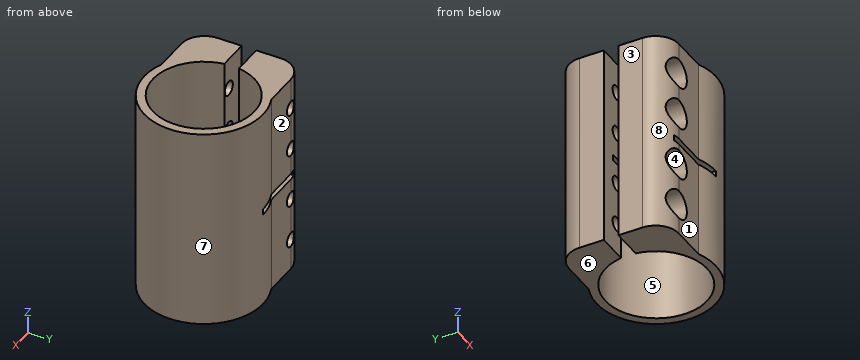
from build123d import *

# Parameters (mm, degrees)
F1_DEPTH       = 35
F3_D           = 5
F3_START       = 1.7550021
F3_CBORE_D     = 10
F3_CBORE_DEPTH = 8
F4_W           = 22.4
F4_H           = 2
F5_DEPTH       = 25


with BuildPart() as f1:
    # F0 (on Top) → F1 (new body, symmetric)
    with BuildSketch(Plane.XY):
        with BuildLine():
            ThreePointArc((-17.3192642082, 2.5086026559), (17.5, 0), (-17.3192642082, -2.5086026559))
            Line((-17.3192642082, -2.5086026559), (-28.1192642082, -2.5086026559))
            Line((-28.1192642082, -2.5086026559), (-28.1192642082, -10.9086026559))
            ThreePointArc((-28.1192642082, -10.9086026559), (-25.7761184577, -16.5654569054), (-20.1192642082, -18.9086026559))
            Line((-20.1192642082, -18.9086026559), (-7.9192642082, -18.9086026559))
            ThreePointArc((-7.9192642082, -18.9086026559), (20.5, 0), (-7.9192642082, 18.9086026559))
            Line((-7.9192642082, 18.9086026559), (-20.1192642082, 18.9086026559))
            ThreePointArc((-20.1192642082, 18.9086026559), (-25.7761184577, 16.5654569054), (-28.1192642082, 10.9086026559))
            Line((-28.1192642082, 10.9086026559), (-28.1192642082, 2.5086026559))
            Line((-28.1192642082, 2.5086026559), (-17.3192642082, 2.5086026559))
        make_face()
    extrude(amount=F1_DEPTH, both=True)

    # F3 (through all)
    # its depths count from where the whole tool has entered the part; down to there all is cleared
    with Locations(Plane.XZ.offset(18.9086026559).offset(-F3_START)):
        with Locations((-20.1192642082, 24.25), (-20.1192642082, 9.25), (-20.1192642082, -9.25), (-20.1192642082, -24.25)):
            CounterBoreHole(F3_D / 2, F3_CBORE_D / 2, F3_CBORE_DEPTH)

    # F4 (on Front) → F5 (cut, symmetric)
    with BuildSketch(Plane.XZ):
        with Locations((-11.2, -1)):
            Rectangle(F4_W, F4_H)
    extrude(amount=F5_DEPTH, both=True, mode=Mode.SUBTRACT)


solid = f1.part
Source: CAD feature listing. Evaluate the final solid. Frame: model axes, mm. Face numbers are marked on the shaded views. A direction names the side the tool comes from. Round coordinates to 2 decimals unless told otherwise and drop trailing zeros. Loops run counter-clockwise (first coordinate to the right, second up) from the corner with the lowest first, then second, coordinate; pieces in that order, holes last.
Q1. Ray query, line 1 (Y direction, x = 0, z = 26.5); line 2 (Z direction, x = -4, y = 19); line 3 (X direction, y = -15, z = -9). Return the intervals inside material, ascending.
Q2. Mould query, pull axis X, two halves, no side actions, for the marked faces 5, 6, 7 and 8. Classes: pulls with the +X half, pulls with the -X half, needs draft (parallel to the pull), parting line crosses it, or undercut.
Q3. Section B-B, the plane z = -10.5. Return loops of the section in (x, y), plus the area to 3 significant figures.
Q4. Access query for the marked faces 1, 2, 3 and 4. Directions: +Z, -Z, +X, -X, +Y, -Y. A direction counts if a zero-diameter tool reaches every point of the face in a straight line with its end or side. Return the directions, or none.
Q5. Section D-D, the plane x = 15.5. Return loops of the section in (y, z).
Q6. First-contact query: P1, Ø8, axis at x = -20.12, z = 24.25, coming from the -Y side; P2, Ø10, axis at x = -10, y = -0.5, coming from the +Z side; P3, Ø3, axis at x = -4.5, z = -23.5, coming from the -Y side; P4, Ø8, axis at x = -20.12, z = 9.25, coming from the +Y side. Flat tips, straight axial feed; report the tip coordinate or a pass-through.
Q7. Section C-C, the plane x = -4. Return loops of the section in (y, z).
Q8. Section A-A, the plane y = -12.5. Return loops of the section in (x, z).
Solutions:
1. line 1: y = -20.5 to -17.5, 17.5 to 20.5
1. line 2: z = -35 to -2, 0 to 35
1. line 3: x = -26.99 to -25.11, -15.13 to -9.01, 9.01 to 13.97
2. face 5: undercut
2. face 6: needs draft
2. face 7: parting line crosses it
2. face 8: pulls with the -X half
3. outline: (-28.12, -10.91) arc R8 ccw to (-24.96, -17.28) - (-24.96, -9.15) - (-22.28, -9.15) - (-22.28, -2.51) - (-28.12, -2.51) - close; (-28.12, 2.51) - (-22.28, 2.51) - (-22.28, 18.61) arc R8 ccw to (-28.12, 10.91) - close; (-17.95, -9.15) - (-15.28, -9.15) - (-15.28, -18.91) - (-7.92, -18.91) arc R20.5 ccw (long way) to (-7.92, 18.91) - (-17.95, 18.91) - (-17.95, 2.51) - (-17.32, 2.51) arc R17.5 cw (long way) to (-17.32, -2.51) - (-17.95, -2.51) - close
3. area: 506 mm2
4. face 1: +Z, -Z, -X, -Y
4. face 2: +Z, -Z, -X, +Y
4. face 3: +Z, -Z, -X, +Y, -Y
4. face 4: -Y
5. outline: (-13.42, -35) - (-8.12, -35) - (-8.12, 35) - (-13.42, 35) - close; (8.12, -35) - (13.42, -35) - (13.42, 35) - (8.12, 35) - close
6. P1: stops at y = -9.15
6. P2: passes through
6. P3: stops at y = -20.28
6. P4: stops at y = 18.91
7. outline: (-20.11, -35) - (-17.04, -35) - (-17.04, -2) - (-20.11, -2) - close; (-20.11, 0) - (-17.04, 0) - (-17.04, 35) - (-20.11, 35) - close; (17.04, -35) - (20.11, -35) - (20.11, -2) - (17.04, -2) - close; (17.04, 0) - (20.11, 0) - (20.11, 35) - (17.04, 35) - close
8. outline: (-27.96, -35) - (-12.25, -35) - (-12.25, -2) - (-22.4, -2) - (-22.4, 0) - (-12.25, 0) - (-12.25, 35) - (-27.96, 35) - close; (12.25, -35) - (16.25, -35) - (16.25, 35) - (12.25, 35) - close; hole circle Ø10 at (-20.12, -24.25); hole circle Ø10 at (-20.12, -9.25); hole circle Ø10 at (-20.12, 9.25); hole circle Ø10 at (-20.12, 24.25)
